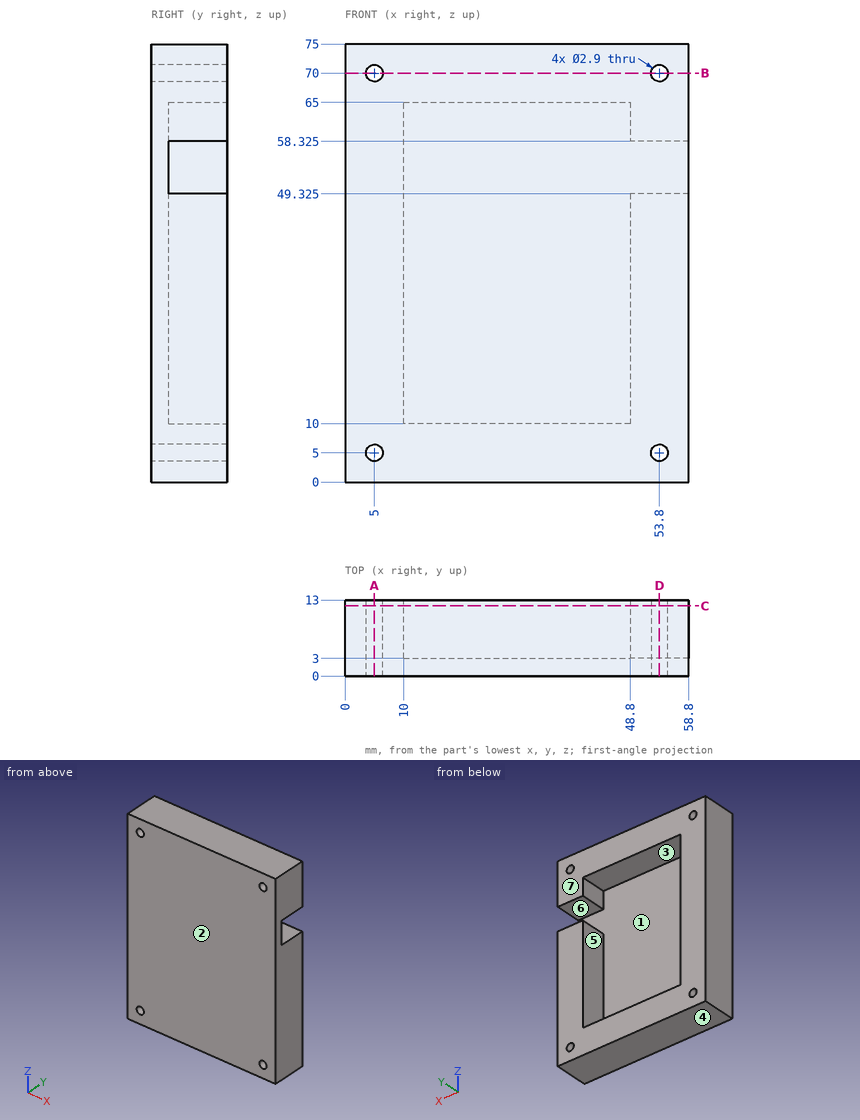
Print and shaded views of the part. All mm, measured from the part's lowest x, y and z. A direction names the side the tool comes from. Round coordinates to 2 decimals unless told otherwise and drop trailing zeros. Write each loop counter-clockwise with the first axis right and the second up, starting at its lowest first coordinate (ties: lowest second). Pieces come first, ordered by that corner, then holes. Notation, with made-up numbers: (29, 32.5) -> (79, 32.5) arc R15 cw to (79, 49.5) -> close; hole circle Ø11 at (28.25, 85.5). An arc over 180 degrees is marked (long way). Answer in a Markdown table with one row per item. Add a question column.
Item 1: Drop a flat-ended pin along its axis: pin 1 Ø5 at (x, y) = (37, 6) entering from -Z. Give the stop position or say it passes through.
Item 2: Which spindle directions (+Z, -Z, +X, -X, +Y, -Y) get a long thin tool onto all of the face, cutting with end or side? Do the marked faces 5, 6 and 7. Say none if no direction does.
Item 3: Saw through at A-A, the plane x = 5. Write the cut outline in (y, z).
Item 4: Saw through at D-D, the plane x = 53.8. Write the cut outline in (y, z) (3 decimals).
Item 5: Saw through at C-C, the plane y = 12. Write the cut outline in (x, z) (3 decimals).
Item 6: Drill centre lines: line 1 (X direction, y = 6.5, z = 5); line 2 (Z direction, x = 53.8, y = 7) (3 decimals); line 3 (X direction, y = 8.25, z = 61.5). Where is each one in solid material? Low to high. Write a range as from..to.
Item 7: Mould opens along Z. For the marked faces 1, 2, 3 and 4 say: pulls with the +Z half, pulls with the -Z half, needs draft (parallel to the pull), parting line crosses it, or undercut.
Item 8: Saw through at B-B, the plane z = 70. Write the cut outline in (x, y), then the cut area to 3 significant figures.
Findings below:
| question | item | result |
|---|---|---|
| 1 | pin 1 | stops at z = 0 |
| 2 | face 5 | +Y |
| 2 | face 6 | +X, +Y |
| 2 | face 7 | +Z, -Z, +X, -X, +Y |
| 3 | outline | (0, 0) -> (13, 0) -> (13, 3.55) -> (0, 3.55) -> close; (0, 6.45) -> (13, 6.45) -> (13, 68.55) -> (0, 68.55) -> close; (0, 71.45) -> (13, 71.45) -> (13, 75) -> (0, 75) -> close |
| 4 | outline | (0, 0) -> (13, 0) -> (13, 3.55) -> (0, 3.55) -> close; (0, 6.45) -> (13, 6.45) -> (13, 49.325) -> (3, 49.325) -> (3, 58.325) -> (13, 58.325) -> (13, 68.55) -> (0, 68.55) -> close; (0, 71.45) -> (13, 71.45) -> (13, 75) -> (0, 75) -> close |
| 5 | outline | (0, 0) -> (58.8, 0) -> (58.8, 49.325) -> (48.8, 49.325) -> (48.8, 10) -> (10, 10) -> (10, 65) -> (48.8, 65) -> (48.8, 58.325) -> (58.8, 58.325) -> (58.8, 75) -> (0, 75) -> close; hole circle Ø2.9 at (5, 5); hole circle Ø2.9 at (5, 70); hole circle Ø2.9 at (53.8, 5); hole circle Ø2.9 at (53.8, 70) |
| 6 | line 1 | x = 0..3.55, 6.45..52.35, 55.25..58.8 |
| 6 | line 2 | z = 0..3.55, 6.45..49.325, 58.325..68.55, 71.45..75 |
| 6 | line 3 | x = 0..10, 48.8..58.8 |
| 7 | face 1 | undercut |
| 7 | face 2 | needs draft |
| 7 | face 3 | undercut |
| 7 | face 4 | pulls with the -Z half |
| 8 | outline | (0, 0) -> (3.55, 0) -> (3.55, 13) -> (0, 13) -> close; (6.45, 0) -> (52.35, 0) -> (52.35, 13) -> (6.45, 13) -> close; (55.25, 0) -> (58.8, 0) -> (58.8, 13) -> (55.25, 13) -> close |
| 8 | area | 689 mm^2 |
